Here's the drawing with two shaded views (mm, measured from the low corner). I have some questions. Give positions to 0.01 mm unless a question says otherwise; leave off trailing zeros. Loops run counter-clockwise (first coordinate to the right, second up) from the corner with the lowest first, then second, coordinate; pieces in that order, holes last.
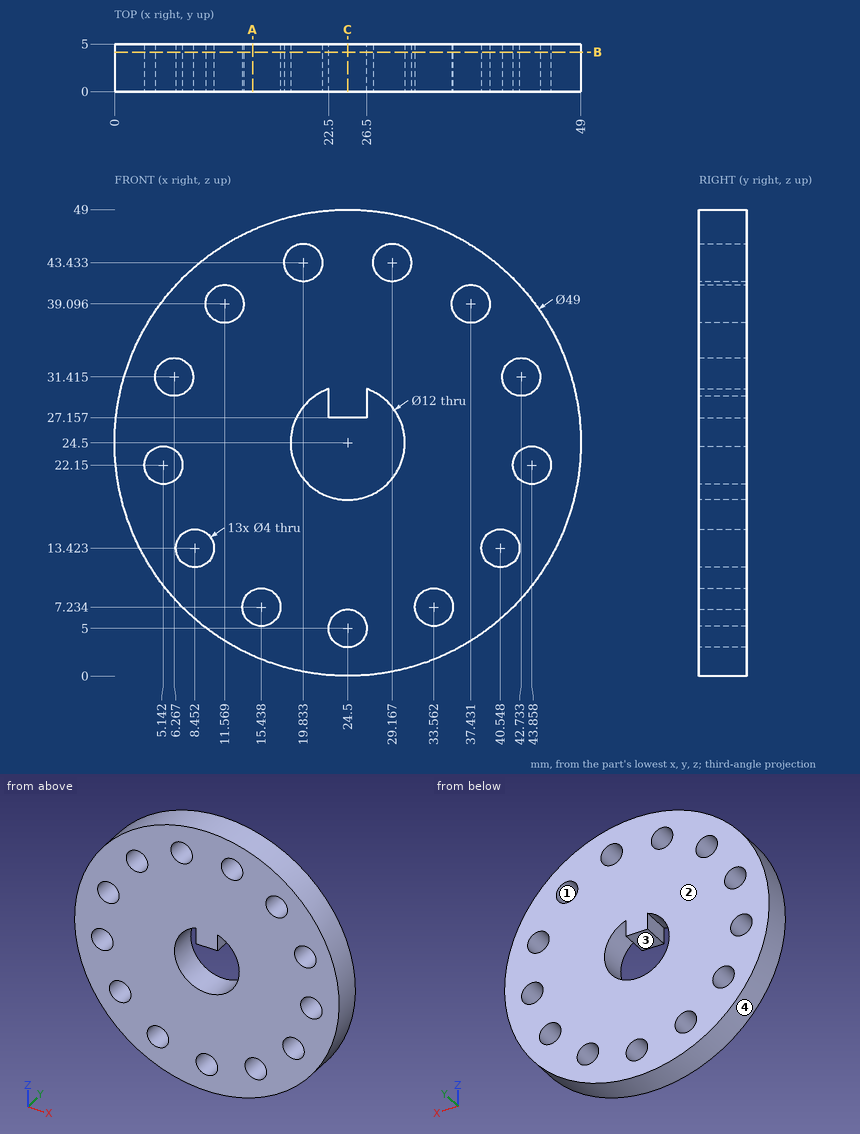
(1) Will these pins go through, and if not, where does the flat tip stop? P1, Ø1.5, axis at y = 3, z = 25.5, coming from the -X side; P2, Ø1.5, axis at y = 2.5, z = 28, coming from the +X side (1 decimal); P3, Ø3.5, axis at x = 15.44, z = 7.23, coming from the +Y side; P4, Ø1, axis at x = 14, y = 4, coming from the +Z side.
Returned:
P1: stops at x = 0
P2: stops at x = 48.8
P3: passes through
P4: stops at z = 46.87
(2) Thinking about a two-plate mould opening in Z: for the marked faces 1, 2, 3 and 4, which applies, pulls with the +Z half, pulls with the -Z half, needs draft (parallel to the pull), parting line crosses it, or undercut?
Returned:
face 1: undercut
face 2: needs draft
face 3: undercut
face 4: parting line crosses it
(3) Suppose I cut it at C-C on x = 24.5. List the corners of the cut face in (y, z) for me, plus the area to 3 significant figures.
Returned:
outline: (0, 0) - (5, 0) - (5, 3) - (0, 3) - close; (0, 7) - (5, 7) - (5, 18.5) - (0, 18.5) - close; (0, 27.16) - (5, 27.16) - (5, 49) - (0, 49) - close
area: 182 mm2
(4) Suppose I cut it at A-A on x = 14.5. List the corners of the cut face in (y, z) for me.
Returned:
outline: (0, 2.13) - (5, 2.13) - (5, 5.47) - (0, 5.47) - close; (0, 9) - (5, 9) - (5, 46.87) - (0, 46.87) - close
(5) Suppose I cut it at B-B on y = 4.15. Give the number of separate pieces and of enclosed holes in the cut face, plus the area to 3 significant figures.
Returned:
separate pieces: 1
enclosed holes: 14
area: 1,620 mm2
(6) Please list where these lines run through material, in increasing order: probe 1 along X at (y, z) = (1.6, 14.5) (1 decimal); probe 2 along X at (y, z) = (2.5, 40.5) (1 decimal); probe 3 along Z at (x, y) = (43.5, 1.2) (1 decimal).
Returned:
probe 1: x = 2.1 to 6.8, 10.1 to 38.9, 42.2 to 46.9
probe 2: x = 5.9 to 10.1, 13 to 36, 38.9 to 43.1
probe 3: z = 9 to 20.2, 24.1 to 29.6, 33.3 to 40
